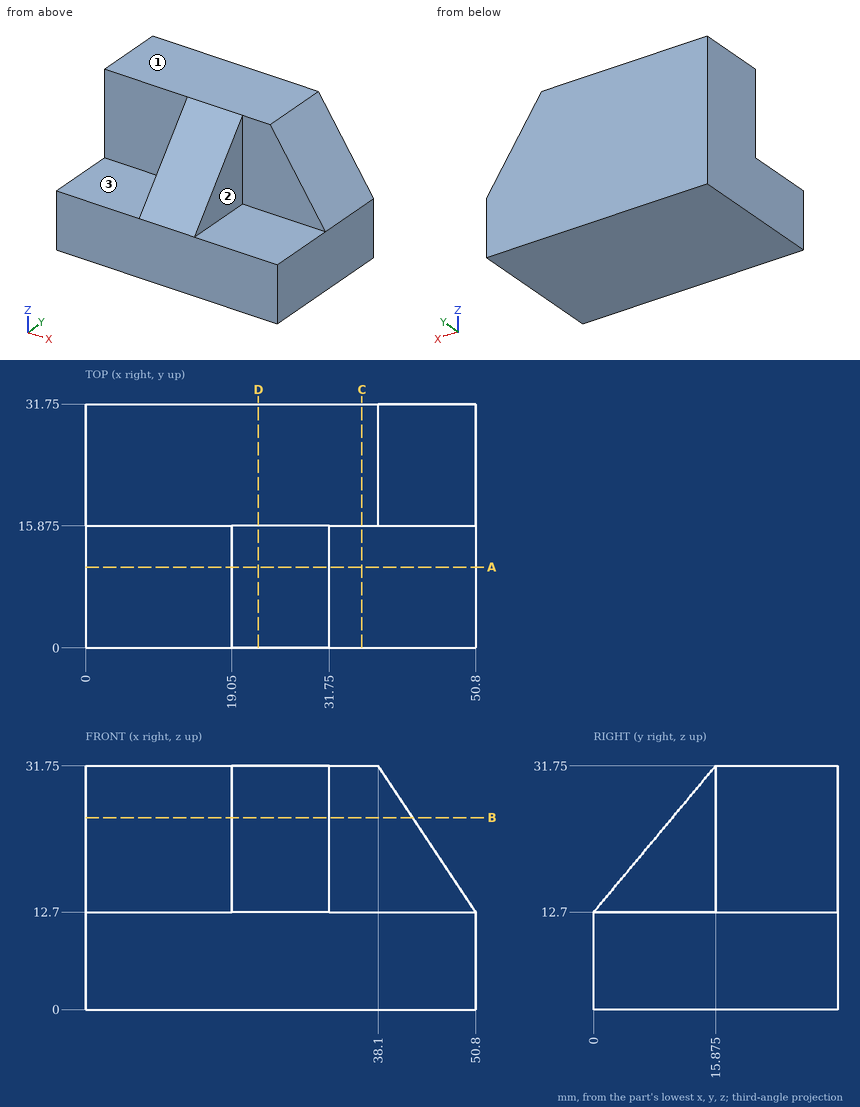
Verification items for this drawing (mm, ordinates from the low corner). A direction names the side the tool comes from. Round coordinates to 2 decimals unless told otherwise and drop trailing zeros. Write each loop counter-clockwise with the first axis right and the second up, starting at its lowest first coordinate (ties: lowest second). Pieces come first, ordered by that corner, then holes. Notation, with made-up numbers: (30.5, 14.25) - (72.5, 14.25) arc R14 ccw to (72.5, 29.25) - close; hole circle Ø2 at (-13.5, 49). An arc over 180 degrees is marked (long way). One line per item, written item: value.
1. Scan lines: L1, parallel to X at y = 11, z = 17; L2, parallel to Z at x = 44, y = 3; L3, parallel to Y at x = 13, z = 21 (3 decimals). Record each from-to range of solid material in increasing order.
The answers:
L1: x = 19.05 to 31.75
L2: z = 0 to 12.7
L3: y = 15.875 to 31.75
2. Cross-section at B-B on z = 25. Record the boundary of the cut face in (x, y) (3 decimals).
The answers:
outline: (0, 15.875) - (19.05, 15.875) - (19.05, 10.25) - (31.75, 10.25) - (31.75, 15.875) - (42.6, 15.875) - (42.6, 31.75) - (0, 31.75) - close
3. Cross-section at D-D on x = 22.5. Record the boundary of the cut face in (y, z) (3 decimals), and give its area (3 significant figures).
The answers:
outline: (0, 0) - (31.75, 0) - (31.75, 31.75) - (15.875, 31.75) - (0, 12.7) - close
area: 857 mm^2
4. Depth check by flat-ended pin: pin 1 Ø3 at (y, z) = (10.5, 22.5) entering from +X; pin 2 Ø10 at (y, z) = (17, 17.5) entering from +X; pin 3 Ø3 at (x, y) = (45.5, 17.5) entering from +Z; pin 4 Ø2 at (x, z) = (14, 20.5) entering from -Y (3 decimals). Enter the tip coordinate at first touch or a pass-through.
The answers:
pin 1: stops at x = 31.75
pin 2: stops at x = 50.8
pin 3: stops at z = 22.9
pin 4: stops at y = 15.875
5. Cross-section at C-C on x = 36. Record the boundary of the cut face in (y, z) (3 decimals), and give its area (3 significant figures).
The answers:
outline: (0, 0) - (31.75, 0) - (31.75, 31.75) - (15.875, 31.75) - (15.875, 12.7) - (0, 12.7) - close
area: 706 mm^2
6. Set-up check for the marked faces 1, 2 and 3: record each of +Z, -Z, +X, -X, +Y, -Y from which the full face is reachable in a straight line by a thin tool's end or side.
The answers:
face 1: +Z, +X, -X, +Y, -Y
face 2: +Z, +X, -Y
face 3: +Z, -X, -Y
7. Cross-section at A-A on y = 10.5. Record the boundary of the cut face in (x, z).
The answers:
outline: (0, 0) - (50.8, 0) - (50.8, 12.7) - (31.75, 12.7) - (31.75, 25.3) - (19.05, 25.3) - (19.05, 12.7) - (0, 12.7) - close
